from build123d import *

# Parameters (mm, degrees)
CHAFL_N1_SIZE         = 0.5
CORTAR_EXTRUIR1_REACH = 67.138
CORTAR_EXTRUIR2_START = -48.6
CORTAR_EXTRUIR2_DEPTH = 12


with BuildPart() as part:
    # Croquis1 → Revolución1 (revolve)
    with BuildSketch(Plane(origin=(0, 0, 0), x_dir=(-1, 0, 0), z_dir=(0, 1, 0)), mode=Mode.PRIVATE) as revoluci_n1_sk:
        Polygon((-32.5, 0), (-32.5, 3), (-20.7, 3), (-20.7, 2.85), (-19.9, 2.85), (-19.9, 3), (26.9, 3), (26.9, 2.85), (27.7, 2.85), (27.7, 3), (32.5, 3), (32.5, 0), align=None)
    revolve(revoluci_n1_sk.sketch.rotate(Axis((32.5, 0, 0), (-1, 0, 0)), 180), axis=Axis((32.5, 0, 0), (-1, 0, 0)))

    # Chaflán1
    chafl_n1_edges = [part.edges().sort_by_distance(p)[0] for p in [
        (32.5, 0, 3),
        (-32.5, 0, 3),
    ]]
    chamfer(chafl_n1_edges, length=CHAFL_N1_SIZE)

    # Cortar-Extruir1: up to this face of the body (flat: up to its plane)
    cortar_extruir1_end = Plane(part.part.faces().sort_by_distance((19.9, 0, 2.934852814))[0])
    # Croquis2 → Cortar-Extruir1 (cut, up to the picked face)
    with BuildSketch(Plane.YZ.offset(32.5), mode=Mode.PRIVATE) as cortar_extruir1_sk1:
        with BuildLine():
            Line((1.658312395, 2.5), (-1.658312395, 2.5))
            ThreePointArc((-1.658312395, 2.5), (0, 3), (1.658312395, 2.5))
        make_face()
    cortar_extruir1_tool1 = split(extrude(cortar_extruir1_sk1.sketch, amount=-CORTAR_EXTRUIR1_REACH, mode=Mode.PRIVATE), bisect_by=cortar_extruir1_end, keep=Keep.BOTH, mode=Mode.PRIVATE)
    add(cortar_extruir1_tool1.solids().sort_by(Axis((32.5, 0, 2.701501), (-1, 0, 0)))[0], mode=Mode.SUBTRACT)

    # Croquis2<2> → Cortar-Extruir2 (cut)
    with BuildSketch(Plane.YZ.offset(32.5).offset(CORTAR_EXTRUIR2_START)):
        with BuildLine():
            Line((1.658312395, 2.5), (-1.658312395, 2.5))
            ThreePointArc((-1.658312395, 2.5), (0, 3), (1.658312395, 2.5))
        make_face()
    extrude(amount=CORTAR_EXTRUIR2_DEPTH, mode=Mode.SUBTRACT)


solid = part.part
Input: part model. Units: mm. Frame: model coordinates. A direction names the side the tool comes from. Coordinates: 2 decimals unless noted, no trailing zeros. Loops run counter-clockwise (first coordinate to the right, second up) from the corner with the lowest first, then second, coordinate; pieces in that order, holes last.
Q1. Material intervals for line 1 (X direction, y = 2.6, z = 1.25); line 2 (Y direction, x = -21, z = 2.5); line 3 (Z direction, x = 25, y = 0.9), sorted ascending.
Q2. Contact query for flat-ended pins moving along their axis: pin 1 (1 mm diameter, centred on x = 24, y = 0.5, fed in from +Z); pin 2 (2 mm diameter, centred on x = 17, y = 2, fed in from +Z). Output: stop coordinate, or through.
Q3. Cut plane A-A (x = -5.5). Output: boundary loops of the cut face in (y, z).
Q4. Draft query along X for faces 1 (the face through (20.294, 0.105, -2.848)), 2 (the face through (32.5, 0, 0)), 3 (the face through (-29.88, -0.9, -2.86)), 4 (the face through (-27.31, 2.78, 0.62)). Return one class per face: +X half, -X half, draft (parallel to the pull), parting line (faces both ways), or undercut.
Q5. Cut plane B-B (x = 4.5). Output: boundary loops of the cut face in (y, z).
Q6. Set-up query: faces 5 (the face through (-10, 0, 2.5)), 6 (the face through (26, 0, 2.5)), 7 (the face through (-32.5, 0, 0)), 8 (the face through (-3.83, -0.9, -2.86)), 9 (the face through (19.9, 0, 2.7)). Return all of +Z, -Z, +X, -X, +Y, -Y with unobstructed straight access to the full face (end or side cutting, diameter ignored); none if empty.
Working result:
1. line 1: x = -32.12 to -27.7, -26.9 to 19.9, 20.7 to 32.12
1. line 2: y = -1.66 to 1.66
1. line 3: z = -2.86 to 2.5
2. pin 1: stops at z = 2.5
2. pin 2: stops at z = 2.83
3. outline: (-1.66, 2.5) arc R3 ccw (long way) to (1.66, 2.5) - close
4. face 1: undercut
4. face 2: +X half
4. face 3: draft
4. face 4: undercut
5. outline: circle Ø6 at (0, 0)
6. face 5: +Z, +Y, -Y
6. face 6: +Z, +X, +Y, -Y
6. face 7: +Z, -Z, -X, +Y, -Y
6. face 8: +X, -X
6. face 9: none
